Check sheet for the modelled part. Datum: model origin and axes. Units: mm. Face numbers are marked on the shaded views. A direction names the side the tool comes from. Round coordinates to 2 decimals unless told otherwise and drop trailing zeros. Order: outer loops, then holes, each group sorted by start corner. A loop starts at its lowest first (then second) coordinate and runs counter-clockwise, first axis right, second up. Notation, with made-up numbers: (64.5, 82.25) -> (103.5, 82.25) arc R14 cw to (103.5, 87.25) -> close; hole circle Ø9 at (-14, 57.25). An arc over 180 degrees is marked (long way). Answer in a Markdown table with one row per item.
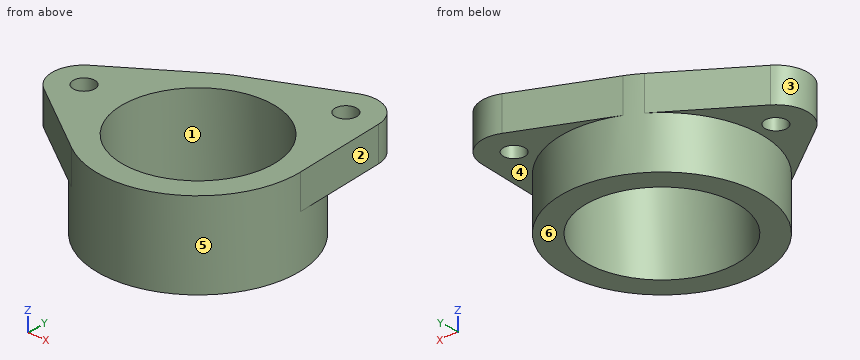
Autodesk Inventor part; units mm, degrees
ref_plane "YZ Plane" through (0, 0, 0) normal (1, 0, 0) x (0, 1, 0)
ref_plane "XZ Plane" through (0, 0, 0) normal (0, 1, 0) x (-1, 0, 0)
ref_plane "XY Plane" through (0, 0, 0) normal (0, 0, 1) x (1, 0, 0)
sketch "スケッチ1" plane through (0, 0, 0) normal (0, 0, 1) x (1, 0, 0)
  circle A0 centre (0, 0) radius 2.25 construction
  circle A1 centre (0, 0) radius 4.35
  circle A2 centre (0, 0) radius 5.75
  circle A3 centre (-6.875, 0) radius 0.625
  circle A4 centre (3.4375, 5.9539) radius 0.625
  circle A5 centre (0, 0) radius 6.875 construction
  circle A6 centre (-6.875, 0) radius 1.825
  circle A7 centre (3.4375, 5.9539) radius 1.825
  line L0 (-7.9169, 1.4983) -> (-3.2827, 4.7208)
  line L1 (-7.9169, -1.4983) -> (-3.2827, -4.7208)
  line L2 (5.2561, 6.1071) -> (5.7297, 0.4825)
  line L3 (-2.447, 5.2033) -> (2.6608, 7.6054)
  line L4 (3.4375, 5.9539) -> (0, 0) construction
  line L5 (0, 0) -> (-6.875, 0) construction
  circle A8 centre (0, 0) radius 4.25
  circle A9 centre (0, 0) radius 4.25
  point P0 (3.9306, 4.1968)
  point P1 (1.6692, 5.5024)
  point P2 (-5.5998, 1.3056)
  point P3 (-5.5998, -1.3056)
  dimension "d2" = 4.5
  dimension "d5" = 1.25
  dimension "d6" = 1.25
  dimension "d7" = 1.2
  dimension "d8" = 1.2
  dimension "d9" = 0.5
  dimension "d18" = 120
  dimension "d22" = 13.75
  dimension "d23" = 8.5
  dimension "d25" = 8.5
  dimension "d26" = 1.5
  dimension "d27" = 0.1
extrude "押し出し1" add sketch "スケッチ1" against normal blind 5 contours A2 A6 A7 | A7 A2 | A2 A6 picked at (2.6949, 4.8059) picked at (-5.5055, 0)
extrude "押し出し3" add sketch "スケッチ1" against normal blind 2 contours L1 A6 A2 | A6 A2 | A6 L0 A2 picked at (-5.951, -0.7528)
extrude "押し出し4" add sketch "スケッチ1" against normal blind 2 contours A2 A7 L2 | A2 A7 | A2 L3 A7 picked at (3.6121, 4.7707)
equation "\"d6\" = d5"
equation "\"d8\" = d7"
properties part number "motorauxiliary"
Item 1: Depth check by flat-ended pin: P1, Ø1.5, axis at x = 4, z = -3.5, coming from the -Y side; P2, Ø1, axis at x = 4, z = -1, coming from the -Y side; P3, Ø3, axis at y = 5, z = -1, coming from the +X side. Enter the tip coordinate at first touch or a pass-through.
Result sheet:
| item | result |
|---|---|
| P1 | stops at y = -4.74 |
| P2 | stops at y = -4.56 |
| P3 | stops at x = 5.48 |
Item 2: Set-up check for the marked faces 5 and 6: record each of +Z, -Z, +X, -X, +Y, -Y from which the full face is reachable in a straight line by a thin tool's end or side.
Result sheet:
| item | result |
|---|---|
| face 5 | -Z |
| face 6 | -Z, +X, -X, +Y, -Y |
Item 3: Cross-section at C-C (z = -0.6). State how many separate pieces and enclosed holes the cut face has, and give its area (3 significant figures).
Result sheet:
| item | result |
|---|---|
| separate pieces | 1 |
| enclosed holes | 3 |
| area | 70.2 mm^2 |
Item 4: Cross-section at B-B (y = -2.25). Record the boundary of the cut face in (x, z), and give its area (3 significant figures).
Result sheet:
| item | result |
|---|---|
| outline | (-6.84, -2) -> (-5.29, -2) -> (-5.29, -5) -> (-3.72, -5) -> (-3.72, 0) -> (-6.84, 0) -> close; (3.72, -5) -> (5.29, -5) -> (5.29, 0) -> (3.72, 0) -> close |
| area | 18.8 mm^2 |
Item 5: Mould release check, pull along X, two halves, no side actions. Record for the marked faces 1, 2, 3 and 4: pulls with the +X half, pulls with the -X half, needs draft (parallel to the pull), parting line crosses it, or undercut.
Result sheet:
| item | result |
|---|---|
| face 1 | undercut |
| face 2 | pulls with the +X half |
| face 3 | pulls with the -X half |
| face 4 | needs draft |
Item 6: Cross-section at D-D (x = 0). Record the boundary of the cut face in (y, z), and give its area (3 significant figures).
Result sheet:
| item | result |
|---|---|
| outline | (-5.75, -5) -> (-4.35, -5) -> (-4.35, 0) -> (-5.75, 0) -> close; (4.35, -5) -> (5.75, -5) -> (5.75, -2) -> (6.35, -2) -> (6.35, 0) -> (4.35, 0) -> close |
| area | 15.2 mm^2 |
Item 7: Cross-section at A-A (y = 0). Record the boundary of the cut face in (x, z).
Result sheet:
| item | result |
|---|---|
| outline | (-8.7, -2) -> (-7.5, -2) -> (-7.5, 0) -> (-8.7, 0) -> close; (-6.25, -2) -> (-5.75, -2) -> (-5.75, -5) -> (-4.35, -5) -> (-4.35, 0) -> (-6.25, 0) -> close; (4.35, -5) -> (5.75, -5) -> (5.75, 0) -> (4.35, 0) -> close |
Item 8: Scan lines: line 1 (Y direction, x = 0, z = -2.05); line 2 (Y direction, x = 3, z = -0.65); line 3 (Y direction, x = -1.75, z = -3.3). Record each from-to range of solid material in increasing order. Write a range as [from, to].
Result sheet:
| item | result |
|---|---|
| line 1 | y = [-5.75, -4.35], [4.35, 5.75] |
| line 2 | y = [-4.91, -3.15], [3.15, 5.51], [6.4, 7.73] |
| line 3 | y = [-5.48, -3.98], [3.98, 5.48] |
